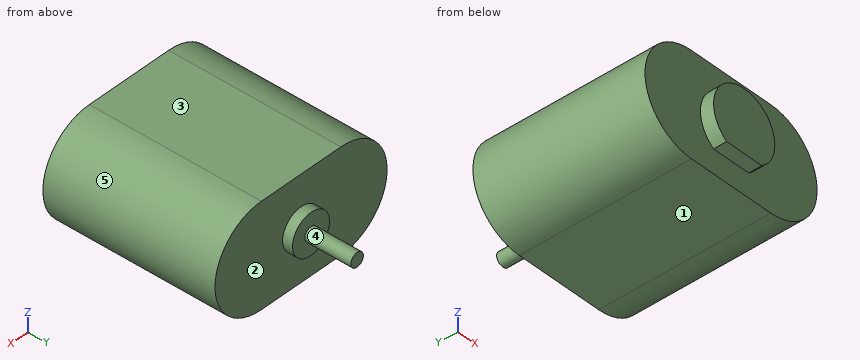
from build123d import *

# Parameters (mm, degrees)
SKETCH1_W           = 12.7
SKETCH1_H           = 14.859
BOSS_EXTRUDE1_DEPTH = 24.9555
SKETCH2_R           = 2.96037
SKETCH2_R_2         = 1.0033
BOSS_EXTRUDE2_DEPTH = 1.4478
SKETCH2_3_R         = 1.0033
BOSS_EXTRUDE3_DEPTH = 8.128
BOSS_EXTRUDE4_DEPTH = 1.905


with BuildPart() as part:
    # Sketch1 → Boss-Extrude1 (new body)
    with BuildSketch(Plane(origin=(0, 0, 0), x_dir=(1, 0, 0), z_dir=(0, 1, 0))):
        with BuildLine():
            Line((-6.35, -7.4295), (-6.35, 7.4295))
            ThreePointArc((-6.35, 7.4295), (-13.7795, 0), (-6.35, -7.4295))
        make_face()
        Rectangle(SKETCH1_W, SKETCH1_H)
        with BuildLine():
            Line((6.35, -7.4295), (6.35, 7.4295))
            ThreePointArc((6.35, 7.4295), (13.7795, 0), (6.35, -7.4295))
        make_face()
    extrude(amount=BOSS_EXTRUDE1_DEPTH)

    # Sketch2 → Boss-Extrude2 (add)
    with BuildSketch(Plane(origin=(0, 24.9555, 0), x_dir=(1, 0, 0), z_dir=(0, 1, 0))):
        with Locations(Location((0, 0, 0), (0, 0, 270))):
            Circle(SKETCH2_R)
        with Locations(Location((0, 0, 0), (0, 0, 270))):
            Circle(SKETCH2_R_2, mode=Mode.SUBTRACT)
    extrude(amount=BOSS_EXTRUDE2_DEPTH)

    # Sketch2_3 → Boss-Extrude3 (add)
    with BuildSketch(Plane(origin=(0, 24.9555, 0), x_dir=(1, 0, 0), z_dir=(0, 1, 0))):
        with Locations(Location((0, 0, 0), (0, 0, 270))):
            Circle(SKETCH2_3_R)
    extrude(amount=BOSS_EXTRUDE3_DEPTH)

    # Sketch3 → Boss-Extrude4 (add)
    with BuildSketch(Plane.XZ):
        with BuildLine():
            Line((-2.815278068, -4.0132), (2.815278068, -4.0132))
            ThreePointArc((2.815278068, -4.0132), (0, 4.9022), (-2.815278068, -4.0132))
        make_face()
    extrude(amount=BOSS_EXTRUDE4_DEPTH)


solid = part.part
The model under review builds one solid part; all positions refer to its coordinate system, in mm. Face numbers are marked on the shaded views. A direction names the side the tool comes from. Round coordinates to 2 decimals unless told otherwise and drop trailing zeros. Order: outer loops, then holes, each group sorted by start corner. A loop starts at its lowest first (then second) coordinate and runs counter-clockwise, first axis right, second up. Notation, with made-up numbers: (-0.5, -40) -> (10.5, -40) arc R25 ccw to (10.5, -13) -> close; hole circle Ø2 at (61.25, 4.25). An arc over 180 degrees is marked (long way). Return JSON: item names as keys, results as strings.
1. Insertion check: P1, Ø1, axis at x = 9, z = -1, coming from the -Y side; P2, Ø4, axis at y = 29, z = -4, coming from the -X side; P3, Ø4.5, axis at x = 4, z = 3, coming from the +Y side; P4, Ø1.5, axis at y = 6.5, z = 3, coming from the -X side. Each pin has a flat end and moves straight along its axis. Give the tip position at first contact, or say it passes through.
Answer block:
{"P1": "stops at y = 0", "P2": "passes through", "P3": "stops at y = 26.4", "P4": "stops at x = -13.43"}
2. Take a section at C-C (y = 14). Write out the cut boundary in (x, z), then the cut area to 3 significant figures.
Answer block:
{"outline": "(-6.35, -7.43) -> (6.35, -7.43) arc R7.43 ccw to (6.35, 7.43) -> (-6.35, 7.43) arc R7.43 ccw to start", "area": "362 mm²"}
3. For L1, parallel to Y at x = 0.5, z = -6; L2, parallel to Y at x = 0, z = 3.5 (1 decimal); L3, parallel to X at y = 23, z = 1.75, list the stretches that pass through material, from the lowest coordinate up. Write a range as [from, to].
Answer block:
{"L1": "y = [0, 24.96]", "L2": "y = [-1.9, 25]", "L3": "x = [-13.57, 13.57]"}
4. Take a section at A-A (z = 0). Write out the cut boundary in (x, y) (1 decimal).
Answer block:
{"outline": "(-13.8, 0) -> (-4.9, 0) -> (-4.9, -1.9) -> (4.9, -1.9) -> (4.9, 0) -> (13.8, 0) -> (13.8, 25) -> (3, 25) -> (3, 26.4) -> (1, 26.4) -> (1, 33.1) -> (-1, 33.1) -> (-1, 26.4) -> (-3, 26.4) -> (-3, 25) -> (-13.8, 25) -> close"}
5. The part is to be moulded in two halves that separate along Z. For the marked faces 1, 2 and 3, say which applies: +Z half, -Z half, draft (parallel to the pull), parting line (faces both ways), or undercut.
Answer block:
{"face 1": "-Z half", "face 2": "draft", "face 3": "+Z half"}
6. For the marked faces 4 and 5, list the 3-axis set-ups (+Z, -Z, +X, -X, +Y, -Y) from which the entire face can be reached by the end or side of a thin tool; tool diameter is ignored.
Answer block:
{"face 4": "+Y", "face 5": "+X, +Y, -Y"}
7. Take a section at B-B (x = 1.5). Write out the cut boundary in (y, z) (1 decimal), then the cut area to 3 significant figures.
Answer block:
{"outline": "(-1.9, -4) -> (0, -4) -> (0, -7.4) -> (25, -7.4) -> (25, -2.6) -> (26.4, -2.6) -> (26.4, 2.6) -> (25, 2.6) -> (25, 7.4) -> (0, 7.4) -> (0, 4.7) -> (-1.9, 4.7) -> close", "area": "395 mm²"}
8. Take a section at D-D (z = 2). Write out the cut boundary in (x, y) (1 decimal).
Answer block:
{"outline": "(-13.5, 0) -> (-4.5, 0) -> (-4.5, -1.9) -> (4.5, -1.9) -> (4.5, 0) -> (13.5, 0) -> (13.5, 25) -> (2.2, 25) -> (2.2, 26.4) -> (-2.2, 26.4) -> (-2.2, 25) -> (-13.5, 25) -> close"}
